from build123d import *

# Parameters (mm, degrees)
SKETCH1_R           = 5.5
BOSS_EXTRUDE1_DEPTH = 4
SKETCH4_R           = 4.15
CUT_EXTRUDE3_DEPTH  = 9.746427842


with BuildPart() as part:
    # Sketch1 → Boss-Extrude1 (new body)
    with BuildSketch(Plane(origin=(0, 0, 0), x_dir=(1, 0, 0), z_dir=(0, 1, 0))):
        with Locations(Location((0, 0, 0), (0, 0, 270))):
            Circle(SKETCH1_R)
    extrude(amount=BOSS_EXTRUDE1_DEPTH)

    # Sketch4 → Cut-Extrude3 (cut, through all)
    with BuildSketch(Plane(origin=(0, 0, 0), x_dir=(1, 0, 0), z_dir=(0, 1, 0))):
        with Locations(Location((0, 0, 0), (0, 0, 270))):
            Circle(SKETCH4_R)
    extrude(amount=CUT_EXTRUDE3_DEPTH, mode=Mode.SUBTRACT)

    # Cut-Sweep1: sweep along a path in Sketch1_2
    with BuildLine(Plane(origin=(0, 0, 0), x_dir=(1, 0, 0), z_dir=(0, 1, 0))) as cut_sweep1_path:
        CenterArc((0, 0), 5.5, 0, 360)
    # Sketch5 → Cut-Sweep1 (sweep, cut)
    with BuildSketch(Plane.XY):
        with BuildLine():
            Line((5.5, 4), (5.5, 0))
            ThreePointArc((5.5, 0), (5.067989981, 2), (5.5, 4))
        make_face()
    sweep(path=cut_sweep1_path.line, mode=Mode.SUBTRACT)


solid = part.part
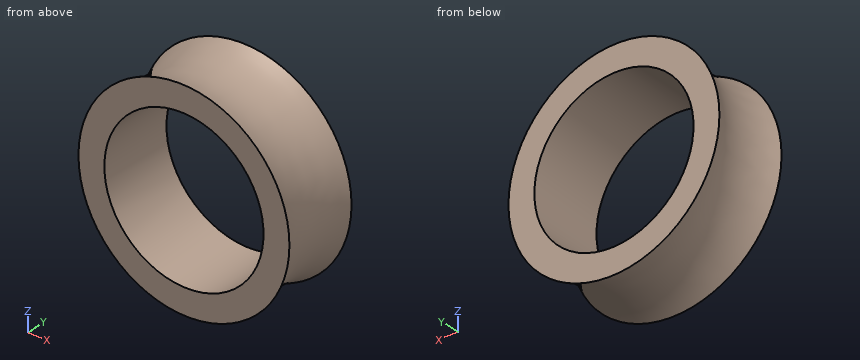
Input: part model. Units: mm. Frame: model coordinates. Give positions to 0.01 mm unless a question says otherwise; leave off trailing zeros. Loops run counter-clockwise (first coordinate to the right, second up) from the corner with the lowest first, then second, coordinate; pieces in that order, holes last. Notation, with made-up numbers: M 31,53.25 L 47,53.25 A27 cw 47,79.25 Z; hole C 85.25,68 d7. An arc over 180 degrees is marked long. Use one line per item in the form item = value.
1. Section query C-C, the plane y = 0.3. Return the cut outline in (x, z).
Numbers:
outline = C 0,0 d10.75; hole C 0,0 d8.3
2. Line query: L1, parallel to X at y = 2, z = 0.75; L2, parallel to X at y = 3, z = 1.75; L3, parallel to Z at x = 2.75, y = 3.15. Output: solid intervals per line, ascending.
Numbers:
L1 = -5.01 to -4.08, 4.08 to 5.01
L2 = -4.87 to -3.76, 3.76 to 4.87
L3 = -4.42 to -3.11, 3.11 to 4.42
3. Section query B-B, the plane z = 0. Return the cut outline in (x, y), and give its area (3 significant figures).
Numbers:
outline = M -5.5,0 L -4.15,0 L -4.15,4 L -5.5,4 A4.85 cw Z; M 4.15,0 L 5.5,0 A4.85 cw 5.5,4 L 4.15,4 Z
area = 8.47 mm²
4. Section query A-A, the plane x = 0. Return the cut outline in (y, z).
Numbers:
outline = M 0,-5.5 A4.85 cw 4,-5.5 L 4,-4.15 L 0,-4.15 Z; M 0,4.15 L 4,4.15 L 4,5.5 A4.85 cw 0,5.5 Z
5. First-contact query: pin 1 (3 mm diameter, centred on x = 3, z = -1, fed in from +Y); pin 2 (3 mm diameter, centred on x = 0, z = -1.5, fed in from +Y). Flat tips, straight axial feed; report the tip coordinate or a pass-through.
Numbers:
pin_1 = 4
pin_2 = through
6. Section query D-D, the plane y = 3.05. Return the cut outline in (x, z), and give its area (3 significant figures).
Numbers:
outline = C 0,0 d10.37; hole C 0,0 d8.3
area = 30.3 mm²
